Verification items for the finished model (mm, model axes). A direction names the side the tool comes from. Give positions to 0.01 mm unless a question says otherwise; leave off trailing zeros. Put each result on its own line as item: value.
from build123d import *

# Parameters (mm, degrees)
EXTRUDE_1_DEPTH     = 15
DRAFT_2_ANGLE       = -20
FILLET_1_R          = 6
FILLET_2_R          = 2
CUT_EXTRUDE_START   = 6
SKETCH_2_R          = 1
CUT_EXTRUDE_1_DEPTH = 59.007812184


with BuildPart() as part:
    # 草图1 → 凸台-拉伸1 (new body)
    with BuildSketch(Plane(origin=(0, 0, 0), x_dir=(1, 0, 0), z_dir=(0, 1, 0))):
        with BuildLine():
            Line((-18.595203517, 39.87754263), (-39.87754263, 18.595203517))
            ThreePointArc((-39.87754263, 18.595203517), (0, -44), (39.87754263, 18.595203517))
            Line((39.87754263, 18.595203517), (18.595203517, 39.87754263))
            ThreePointArc((18.595203517, 39.87754263), (0, 44), (-18.595203517, 39.87754263))
        make_face()
    extrude(amount=EXTRUDE_1_DEPTH)

    # 拔模2
    draft_2_faces = [part.faces().sort_by_distance(p)[0] for p in [
        (29.236373073, 7.5, -29.236373073),
        (0, 7.5, 44),
        (-29.236373073, 7.5, -29.236373073),
        (0, 7.5, -44),
    ]]
    draft(draft_2_faces, Plane(origin=(0, 0, 0), x_dir=(0, 0, -1), z_dir=(0, -1, 0)), DRAFT_2_ANGLE)

    # 圆角1
    fillet_1_edges = [part.edges().sort_by_distance(p)[0] for p in [
        (17.010833705, 7.500497123, -37.601169244),
        (37.601169244, 7.500497123, -17.010833705),
        (-37.601169244, 7.500497123, -17.010833705),
        (-17.010833705, 7.500497123, -37.601169244),
    ]]
    fillet(fillet_1_edges, radius=FILLET_1_R)

    # 圆角2
    fillet_2_edges = [part.edges().sort_by_distance(p)[0] for p in [
        (-35.248872303, 15, -15.340682868),
        (-25.375885761, 15, -25.375885761),
        (-15.340682868, 15, -35.248872303),
        (0, 15, -38.540446486),
        (15.340682868, 15, -35.248872303),
        (25.375885761, 15, -25.375885761),
        (35.248872303, 15, -15.340682868),
        (0, 15, 38.540446486),
    ]]
    fillet(fillet_2_edges, radius=FILLET_2_R)

    # 草图2 → 切除-拉伸1 (cut, through all)
    with BuildSketch(Plane(origin=(0, 0, 0), x_dir=(1, 0, 0), z_dir=(0, 1, 0)).offset(CUT_EXTRUDE_START)):
        with Locations(Location((0, -32.614789591, 0), (0, 0, 270))):
            Circle(SKETCH_2_R)
    extrude(amount=CUT_EXTRUDE_1_DEPTH, mode=Mode.SUBTRACT)


solid = part.part
Q1. Scan lines: line 1 along Z through (x, y) = (0, 13.25); line 2 along Z through (x, y) = (0, 11.75); line 3 along Y through (x, z) = (-16, -34.5). Record each from-to range of solid material in increasing order.
Answers follow:
line 1: z = -39.18 to 31.61, 33.61 to 39.18
line 2: z = -39.72 to 31.61, 33.61 to 39.72
line 3: y = 0 to 14.58
Q2. Go/stop test with flat-tipped pins: pin 1 Ø8 at (y, z) = (12.5, 12) entering from +X; pin 2 Ø6 at (y, z) = (6, -31) entering from -X; pin 3 Ø6 at (x, y) = (1.5, 12.5) entering from -Z. Record where each tip stops, or that it passes through.
Answers follow:
pin 1: stops at x = 39.47
pin 2: stops at x = -27.76
pin 3: stops at z = -40.52
Q3. Set-up check for faces 4 (the face through (27.64, 6.75, -27.36)), 5 (the face through (0.044, 10.437, 31.616)): record each of +Z, -Z, +X, -X, +Y, -Y from which the full face is reachable in a straight line by a thin tool's end or side.
Answers follow:
face 4: -Z, +X, +Y
face 5: +Y
Q4. Release check for a two-part mould opening along Z. For faces 1 (the face through (-27.36, 6.75, -27.64)), 2 (the face through (0, 6, 33)), 3 (the face through (-1, 0, -1)) record: released by +Z, released by -Z, zero draft, split by the parting line, or undercut.
Answers follow:
face 1: released by -Z
face 2: undercut
face 3: zero draft
